Part model, mm, in its own coordinate system. A direction names the side the tool comes from. Give positions to 0.01 mm unless a question says otherwise; leave off trailing zeros. Write each loop counter-clockwise with the first axis right and the second up, starting at its lowest first coordinate (ties: lowest second). Pieces come first, ordered by that corner, then holes. Notation, with made-up numbers: M -19.75,26.5 L 5.25,26.5 A16 ccw 5.25,51.5 Z; hole C 69.25,40.25 d3. An arc over 180 degrees is marked long. Answer as CSV lines item,"result". Start each with the question number.
Item 1: Two-plate mould, pull along X, no slides. Class faces 1 (the flat face through (-47, 431.8, -15)), 2 (the flat face through (-98.552, -281, 9)), 3 (the flat face through (-175.724, 156, 2)), 4 (the flat face through (59.493, 412.483, -15.027)): +X half, -X half, draft (parallel to the pull), parting line (faces both ways), or undercut.
Item 2: Band-saw the part on A-A, the plane y = -132. List the corners of the cut face in (x, z), then the cut area to 3 significant figures.
Item 3: 3-axis set-ups, long thin cutter, end or side, ignore diameter. For faces 5 (the flat face through (-54.696, -389.922, 8.766)), 6 (the flat face through (20.32, -25, 9)), 7 (the flat face through (-59.847, -26, 9)), 8 (the flat face through (-166, 115, 0)): which of +Z, -Z, +X, -X, +Y, -Y reach the whole face in a straight line?
Item 4: Pin check, flat tips, straight feed: pin 1 (8.5 mm diameter, centred on x = -51.5, y = -121, fed in from -Z); pin 2 (19.5 mm diameter, centred on y = -142, z = 8.5, fed in from -X); pin 3 (1 mm diameter, centred on x = -50.5, y = -90.5, fed in from +Z). Stop position of each tip, or through.
Item 5: Wall check: L1, parallel to X at y = 323, z = -13; L2, parallel to X at y = -109, z = 12; L3, parallel to Y at x = -96, z = 2. Give the ranges that are in metal, low to high. Write a range as from..to.
Item 6: Band-saw the part on C-C, the plane y = 114.3. List the corners of the cut face in (x, z), then the cut area to 3 significant figures.
Item 7: Band-saw the part on B-B, the plane y = 323.85. List the corners of the cut face in (x, z).
from build123d import *

# Parameters (mm, degrees)
BOSS_EXTRUDE1_DEPTH   = 17.78
BOSS_EXTRUDE1_2_DEPTH = 17.78
BOSS_EXTRUDE1_3_DEPTH = 17.78
SKETCH2_W             = 254
SKETCH2_H             = 254
BOSS_EXTRUDE2_DEPTH   = 50.8
FILLET1_R             = 25.4
SKETCH3_R             = 25.4
CUT_EXTRUDE1_DEPTH    = 50.8
BOSS_EXTRUDE3_DEPTH   = 30.48
SKETCH5_R             = 38.1
CUT_EXTRUDE2_DEPTH    = 30.48


with BuildPart() as part:
    # Sketch1 → Boss-Extrude1 (new body)
    with BuildSketch(Plane.XY):
        Polygon((0, 0), (20.32, 0), (20.32, -50.8), (24.432509982, -50.8), (24.432509982, -177.8), (20.32, -177.8), (20.32, -381), (10.16, -398.597636205), (0, -381), (0, -177.8), (-4.523490018, -177.8), (-4.523490018, -50.8), (0, -50.8), align=None)
    extrude(amount=BOSS_EXTRUDE1_DEPTH)



with BuildPart() as body_2:
    # Sketch1 → Boss-Extrude1 2 (new body)
    with BuildSketch(Plane.XY):
        Polygon((-59.846980035, -50.8), (-59.846980035, 0), (-39.526980035, 0), (-39.526980035, -50.8), (-35.003490018, -50.8), (-35.003490018, -177.8), (-39.526980035, -177.8), (-39.526980035, -381), (-49.686980035, -398.597636205), (-59.846980035, -381), (-59.846980035, -177.8), (-63.959490018, -177.8), (-63.959490018, -50.8), align=None)
    extrude(amount=BOSS_EXTRUDE1_2_DEPTH)


with BuildPart() as body_3:
    # Sketch1 → Boss-Extrude1 3 (new body)
    with BuildSketch(Plane.XY):
        Polygon((-118.872, -381), (-108.712, -398.597636205), (-98.552, -381), (-98.552, -177.8), (-94.439490018, -177.8), (-94.439490018, -50.8), (-98.552, -50.8), (-98.552, 0), (-118.872, 0), (-118.872, -50.8), (-123.395490018, -50.8), (-123.395490018, -177.8), (-118.872, -177.8), align=None)
    extrude(amount=BOSS_EXTRUDE1_3_DEPTH)


with BuildPart() as part_1:
    add(part.part)

    add(body_2.part)  # Boss-Extrude2 merges body 2

    add(body_3.part)  # Boss-Extrude2 merges body 3
    # Sketch2 → Boss-Extrude2 (add)
    with BuildSketch(Plane.XY):
        with Locations((-48.724161458, 127)):
            Rectangle(SKETCH2_W, SKETCH2_H)
    extrude(amount=BOSS_EXTRUDE2_DEPTH)

    # Fillet1
    fillet1_edges = [part_1.edges().sort_by_distance(p)[0] for p in [
        (-48.724161458, 254, 50.8),
    ]]
    fillet(fillet1_edges, radius=FILLET1_R)

    # Sketch3 → Cut-Extrude1 (cut)
    with BuildSketch(Plane.XY.offset(50.8)):
        with Locations((-175.724161458, 114.3)):
            Circle(SKETCH3_R)
        with Locations((78.275838542, 114.3)):
            Circle(SKETCH3_R)
    extrude(amount=-CUT_EXTRUDE1_DEPTH, mode=Mode.SUBTRACT)

    # Sketch4 → Boss-Extrude3 (add)
    with BuildSketch(Plane(origin=(0, 0, 0), x_dir=(-1, 0, 0), z_dir=(0, 0, -1))):
        Polygon((-78.275838542, 393.7), (-40.175838542, 431.8), (137.624161458, 431.8), (175.724161458, 393.7), (175.724161458, 0), (-78.275838542, 0), align=None)
    extrude(amount=BOSS_EXTRUDE3_DEPTH)

    # Sketch5 → Cut-Extrude2 (cut)
    with BuildSketch(Plane.XY):
        with Locations((-48.724161458, 323.85)):
            Circle(SKETCH5_R)
    extrude(amount=-CUT_EXTRUDE2_DEPTH, mode=Mode.SUBTRACT)


solid = part_1.part
Output:
1,face 1,"draft"
1,face 2,"undercut"
1,face 3,"-X half"
1,face 4,"+X half"
2,outline,"M -123.4,0 L -94.44,0 L -94.44,17.78 L -123.4,17.78 Z; M -63.96,0 L -35,0 L -35,17.78 L -63.96,17.78 Z; M -4.52,0 L 24.43,0 L 24.43,17.78 L -4.52,17.78 Z"
2,area,"1,540 mm²"
3,face 5,"+Z, -Z, -Y"
3,face 6,"+Z, -Z, +X"
3,face 7,"+Z, -Z"
3,face 8,"+Z, -X"
4,pin 1,"z = 0"
4,pin 2,"x = -123.4"
4,pin 3,"z = 17.78"
5,L1,"-175.72..-86.81, -10.63..78.28"
5,L2,"-123.4..-94.44, -63.96..-35, -4.52..24.43"
5,L3,"-177.8..-50.8, 0..254"
6,outline,"M -175.72,-30.48 L 78.28,-30.48 L 78.28,0 L 52.88,0 L 52.88,50.8 L -150.32,50.8 L -150.32,0 L -175.72,0 Z"
6,area,"18,100 mm²"
7,outline,"M -175.72,-30.48 L -86.82,-30.48 L -86.82,0 L -175.72,0 Z; M -10.62,-30.48 L 78.28,-30.48 L 78.28,0 L -10.62,0 Z"
